```python
from build123d import *

# Parameters (mm, degrees)
SKETCH2_W                    = 464.185
SKETCH2_H                    = 127.5715
BASE_FLANGE1_DEPTH           = 3.175
BOSS_EXTRUDE1_DEPTH          = 3.175
EDGE_FLANGE1_STRIP_W         = 17.24
EDGE_FLANGE1_STRIP_H         = 3.175
EDGE_FLANGE1_STRIP_CUT_DEPTH = 464.185
EDGE_FLANGE1_DEPTH           = 464.185


# Sheet-metal steps are written as plain solids
with BuildPart() as part:
    # Sketch2 → Base-Flange1 (new body)
    with BuildSketch(Plane(origin=(0, 0, 0), x_dir=(1, 0, 0), z_dir=(0, 1, 0))):
        Rectangle(SKETCH2_W, SKETCH2_H)
    extrude(amount=-BASE_FLANGE1_DEPTH)

    # Sketch7 → Boss-Extrude1 (add)
    with BuildSketch(Plane(origin=(0, 0, 0), x_dir=(1, 0, 0), z_dir=(0, 1, 0))):
        Polygon((-232.0925, 63.78575), (232.0925, 63.78575), (232.0925, 152.68575), (-155.8925, 152.68575), (-232.0925, 76.48575), align=None)
    extrude(amount=-BOSS_EXTRUDE1_DEPTH)

    # Edge-Flange1 strip (across the edge) → Edge-Flange1 strip cut (cut)
    with BuildSketch(Plane(origin=(232.0925, -3.175, 66.32575), x_dir=(0, 0, -1), z_dir=(-1, 0, 0))):
        with Locations((-4.445, -1.5875)):
            Rectangle(EDGE_FLANGE1_STRIP_W, EDGE_FLANGE1_STRIP_H)
    extrude(amount=EDGE_FLANGE1_STRIP_CUT_DEPTH, mode=Mode.SUBTRACT)

    # Edge-Flange1 section (across the edge) → Edge-Flange1 (add)
    with BuildSketch(Plane(origin=(232.0925, -3.175, 66.32575), x_dir=(0, 0, -1), z_dir=(-1, 0, 0))):
        with BuildLine():
            Line((0, 1), (0, 15.875))
            Line((0, 15.875), (3.175, 15.875))
            Line((3.175, 15.875), (3.175, 1))
            ThreePointArc((3.175, 1), (3.467893219, 0.292893219), (4.175, 0))
            Line((4.175, 0), (4.175, -3.175))
            ThreePointArc((4.175, -3.175), (1.222829189, -1.952170811), (0, 1))
        make_face()
    extrude(amount=EDGE_FLANGE1_DEPTH)


solid = part.part
```
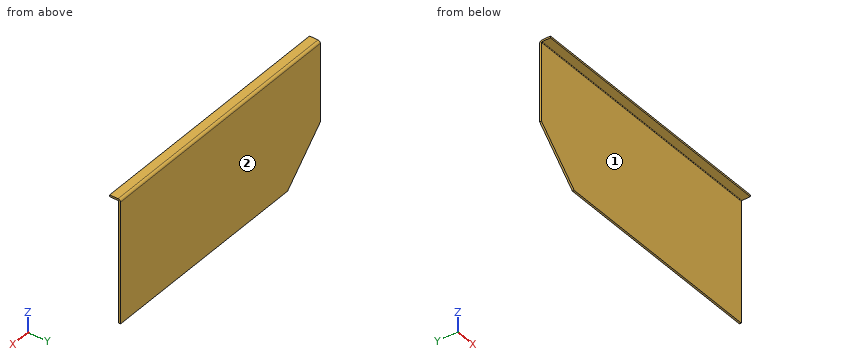
Here's how the part is built. I have some questions about the finished solid (model axes, mm). Face numbers are marked on the shaded views. A direction names the side the tool comes from. Round coordinates to 2 decimals unless told otherwise and drop trailing zeros. Order: outer loops, then holes, each group sorted by start corner. A loop starts at its lowest first (then second) coordinate and runs counter-clockwise, first axis right, second up. Notation, with made-up numbers: (-10.75, 52) -> (37.25, 52) arc R37 ccw to (37.25, 88) -> close; hole circle Ø5 at (46.5, 19.25). An arc over 180 degrees is marked (long way). Use a Markdown table: item, result. Add a question column.
(1) Suppose I cut it at D-D, the plane x = -169. Please give me the cut outline in (y, z) (3 decimals).
(2) Suppose I cut it at A-A, the plane x = 186. Please give me the cut outline in (y, z) (3 decimals).
(3) I need wall thicknesses on line 1 along Y through (x, z) = (53.5, -107) (3 decimals); line 2 along Z through (x, y) = (-146, -12.75); line 3 along X through (y, z) = (-1, -91.5). Which ranges of each line are inside material? Lowest first, please.
(4) For pin 1 Ø10 at (x, y) = (-120.5, -11.5) entering from -Z; pin 2 Ø5 at (x, z) = (166, 13.5) entering from -Y (3 decimals), each with a flat end and sliding along its axis, tell me the tip position at first contact or that it passes through.
(5) For the marked faces 1 and 2, which set-ups out of +Z, -Z, +X, -X, +Y, -Y let a thin tool reach every point of the face, with its end or its side?
(6) Suppose I cut it at B-B, the plane y = -12. Please give me the cut outline in (x, z), and give its area (3 significant figures).
(7) Suppose I cut it at C-C, the plane z = 2.5. Please give me the cut outline in (x, y) (1 decimal).
Verdict:
| question | item | result |
|---|---|---|
| 1 | outline | (-19.05, 63.151) -> (-4.175, 63.151) arc R1 cw to (-3.175, 62.151) -> (-3.175, -139.578) -> (0, -139.578) -> (0, 62.151) arc R4.175 ccw to (-4.175, 66.326) -> (-19.05, 66.326) -> close |
| 2 | outline | (-19.05, 63.151) -> (-4.175, 63.151) arc R1 cw to (-3.175, 62.151) -> (-3.175, -152.686) -> (0, -152.686) -> (0, 62.151) arc R4.175 ccw to (-4.175, 66.326) -> (-19.05, 66.326) -> close |
| 3 | line 1 | -3.175 to 0 |
| 3 | line 2 | 63.15 to 66.33 |
| 3 | line 3 | -217.08 to 232.09 |
| 4 | pin 1 | z = 63.15 |
| 4 | pin 2 | y = -3.175 |
| 5 | face 1 | -Z, +X, -X, -Y |
| 5 | face 2 | +Z, -Z, +X, -X, +Y |
| 6 | outline | (-232.09, 63.15) -> (232.09, 63.15) -> (232.09, 66.33) -> (-232.09, 66.33) -> close |
| 6 | area | 1,470 mm2 |
| 7 | outline | (-232.1, -3.2) -> (232.1, -3.2) -> (232.1, 0) -> (-232.1, 0) -> close |
